Verification items for the finished model (mm, model axes). Face numbers are marked on the shaded views. A direction names the side the tool comes from. Round coordinates to 2 decimals unless told otherwise and drop trailing zeros. Loops run counter-clockwise (first coordinate to the right, second up) from the corner with the lowest first, then second, coordinate; pieces in that order, holes last. Notation, with made-up numbers: (6.25, 77.25) -> (36.25, 77.25) arc R36 cw to (36.25, 113.25) -> close; hole circle Ø4 at (70.25, -3). An arc over 180 degrees is marked (long way). Write item = value, one per line.
```python
from build123d import *

# Parameters (mm, degrees)
SKETCH1_R           = 1.0922
BOSS_EXTRUDE1_DEPTH = 3.175


with BuildPart() as part:
    # Sketch1 → Boss-Extrude1 (new body)
    with BuildSketch(Plane.XY):
        with BuildLine():
            Line((97.519253807, 20.554833153), (97.617319935, 20.554833153))
            ThreePointArc((97.617319935, 20.554833153), (98.725143354, 20.766872021), (99.67636569, 21.373014971))
            ThreePointArc((99.67636569, 21.373014971), (103.892237153, 19.554833153), (99.67636569, 17.736651335))
            ThreePointArc((99.67636569, 17.736651335), (98.725143354, 18.342794285), (97.617319935, 18.554833153))
            Line((97.617319935, 18.554833153), (97.519253807, 18.554833153))
            Line((97.519253807, 18.554833153), (95.269253807, 18.554833153))
            ThreePointArc((95.269253807, 18.554833153), (94.738923721, 18.774503067), (94.519253807, 19.304833153))
            Line((94.519253807, 19.304833153), (94.519253807, 19.804833153))
            ThreePointArc((94.519253807, 19.804833153), (94.738923721, 20.335163239), (95.269253807, 20.554833153))
            Line((95.269253807, 20.554833153), (97.519253807, 20.554833153))
        make_face()
        with Locations((101.392237153, 19.554833153)):
            Circle(SKETCH1_R, mode=Mode.SUBTRACT)
    extrude(amount=BOSS_EXTRUDE1_DEPTH)


solid = part.part
```
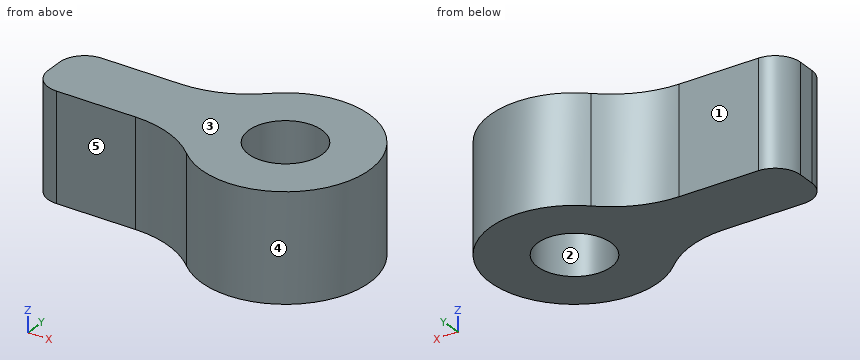
(1) Sectioned sample at D-D, the plane x = 97.5. Record the cut outline in (y, z) (3 decimals).
Filled sheet:
outline = (18.555, 0) -> (20.555, 0) -> (20.555, 3.175) -> (18.555, 3.175) -> close
(2) Set-up check for the marked faces 4 and 5: record each of +Z, -Z, +X, -X, +Y, -Y from which the full face is reachable in a straight line by a thin tool's end or side.
Filled sheet:
face_4 = +Z, -Z
face_5 = +Z, -Z, -X, -Y
(3) Material ranges on probe 1 along Y at (x, z) = (97, 1.3); probe 2 along X at (y, z) = (19.55, 1.3); probe 3 along Y at (x, z) = (101.25, 2.8), recorded low to high. Write a range as from..to.
Filled sheet:
probe_1 = 18.55..20.55
probe_2 = 94.52..100.3, 102.48..103.89
probe_3 = 17.06..18.47, 20.64..22.05
(4) Sectioned sample at B-B, the plane z = 2.6. Record the cut outline in (x, y).
Filled sheet:
outline = (94.52, 19.3) arc R0.75 ccw to (95.27, 18.55) -> (97.62, 18.55) arc R3 cw to (99.68, 17.74) arc R2.5 ccw (long way) to (99.68, 21.37) arc R3 cw to (97.62, 20.55) -> (95.27, 20.55) arc R0.75 ccw to (94.52, 19.8) -> close; hole circle Ø2.18 at (101.39, 19.55)
(5) Draft check along Y on the marked faces 1, 2 and 3. Enter one of: released by +Y, released by -Y, zero draft, split by the parting line, or undercut.
Filled sheet:
face_1 = released by +Y
face_2 = undercut
face_3 = zero draft
(6) Go/stop test with flat-tipped pins: pin 1 Ø1.5 at (x, z) = (97, 2.5) entering from +Y; pin 2 Ø0.7 at (x, z) = (97, 2.5) entering from -Y; pin 3 Ø1 at (x, z) = (100, 0.5) entering from +Y. Record where each tip stops, or that it passes through.
Filled sheet:
pin_1 = 20.56
pin_2 = 18.55
pin_3 = 21.89
(7) Sectioned sample at A-A, the plane y = 19.9. Record the cut outline in (x, z) (3 decimals).
Filled sheet:
outline = (94.525, 0) -> (100.356, 0) -> (100.356, 3.175) -> (94.525, 3.175) -> close; (102.428, 0) -> (103.868, 0) -> (103.868, 3.175) -> (102.428, 3.175) -> close
(8) Sectioned sample at C-C, the plane x = 101.25. Record the cut outline in (y, z) (3 decimals).
Filled sheet:
outline = (17.059, 0) -> (18.472, 0) -> (18.472, 3.175) -> (17.059, 3.175) -> close; (20.638, 0) -> (22.051, 0) -> (22.051, 3.175) -> (20.638, 3.175) -> close
